Verification items for this drawing (mm, ordinates from the low corner). A direction names the side the tool comes from. Round coordinates to 2 decimals unless told otherwise and drop trailing zeros. Order: outer loops, then holes, each group sorted by start corner. A loop starts at its lowest first (then second) coordinate and runs counter-clockwise, first axis right, second up. Notation, with made-up numbers: (7, 7.25) -> (60, 7.25) arc R15 cw to (60, 14.25) -> close; hole circle Ø6 at (7, 24). An arc over 180 degrees is marked (long way). Use a Markdown table: item, result. Add a question column.
Item 1: Sectioned sample at B-B, the plane y = 6.25. State how many separate pieces and enclosed holes the cut face has, and give its area (3 significant figures).
Item 2: Sectioned sample at A-A, the plane x = 27.25. Record the cut outline in (y, z), and give its area (3 significant figures).
Item 3: Sectioned sample at C-C, the plane z = 19.75. Record the cut outline in (x, y).
Item 4: Material ranges on probe 1 along Z at (x, y) = (9, 2.25); probe 2 along X at (y, z) = (5.5, 24) (1 decimal); probe 3 along X at (y, z) = (2.5, 23) (1 decimal), recorded low to high. Write a range as [from, to].
Item 5: Set-up check for the marked faces 5 and 6: record each of +Z, -Z, +X, -X, +Y, -Y from which the full face is reachable in a straight line by a thin tool's end or side.
Item 6: Sectioned sample at D-D, the plane z = 24. Record the cut outline in (x, y) (1 decimal).
Item 7: Gauge pin test, flat ends, axial feed: pin 1 Ø2 at (x, y) = (18, 4) entering from -Z; pin 2 Ø1 at (x, y) = (10.5, 6) entering from -Z; pin 3 Ø3.5 at (x, z) = (19.5, 12) entering from -Y; pin 4 Ø2 at (x, z) = (20.48, 24.5) entering from -Y. Record the tip position at first contact, or that the pin passes through.
Item 8: Mould release check, pull along Z, two halves, no side actions. Record for the marked faces 1, 2, 3 and 4: pulls with the +Z half, pulls with the -Z half, needs draft (parallel to the pull), parting line crosses it, or undercut.
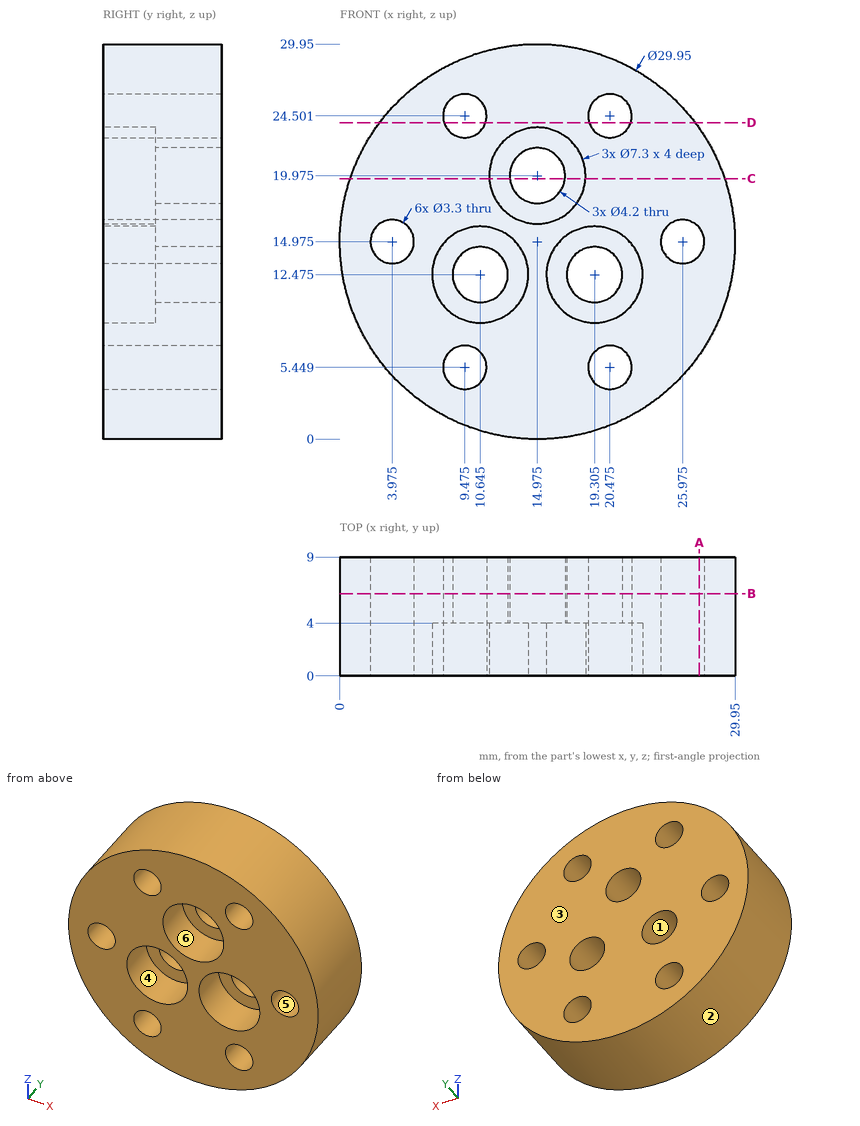
Found:
| question | item | result |
|---|---|---|
| 1 | separate pieces | 1 |
| 1 | enclosed holes | 9 |
| 1 | area | 612 mm2 |
| 2 | outline | (0, 6.4) -> (9, 6.4) -> (9, 13.93) -> (0, 13.93) -> close; (0, 16.02) -> (9, 16.02) -> (9, 23.55) -> (0, 23.55) -> close |
| 2 | area | 136 mm2 |
| 3 | outline | (0.78, 0) -> (11.33, 0) -> (11.33, 4) -> (12.89, 4) -> (12.89, 9) -> (0.78, 9) -> close; (17.06, 4) -> (18.62, 4) -> (18.62, 0) -> (29.17, 0) -> (29.17, 9) -> (17.06, 9) -> close |
| 4 | probe 1 | z = [1.24, 3.87], [7.03, 9.22], [15.73, 22.92], [26.08, 28.71] |
| 4 | probe 2 | x = [3, 7.9], [11, 18.9], [22, 26.9] |
| 4 | probe 3 | x = [2.3, 8.8], [10.2, 12.9], [17, 19.8], [21.2, 27.6] |
| 5 | face 5 | +Y, -Y |
| 5 | face 6 | -Y |
| 6 | outline | (3, 0) -> (7.9, 0) -> (7.9, 9) -> (3, 9) -> close; (11, 0) -> (18.9, 0) -> (18.9, 9) -> (11, 9) -> close; (22, 0) -> (26.9, 0) -> (26.9, 9) -> (22, 9) -> close |
| 7 | pin 1 | stops at z = 0.14 |
| 7 | pin 2 | stops at z = 0.54 |
| 7 | pin 3 | stops at y = 4 |
| 7 | pin 4 | passes through |
| 8 | face 1 | undercut |
| 8 | face 2 | parting line crosses it |
| 8 | face 3 | needs draft |
| 8 | face 4 | undercut |
